The listing builds one solid part. Answer for the finished solid, in the listing's coordinates (mm). Round coordinates to 2 decimals unless told otherwise and drop trailing zeros. Loops run counter-clockwise (first coordinate to the right, second up) from the corner with the lowest first, then second, coordinate; pieces in that order, holes last. Notation, with made-up numbers: M 27.25,22 L 40.25,22 A13 ccw 40.25,47 Z; hole C 34,35 d7. An arc over 180 degrees is marked long. Put each result on its own line as item: value. Start each with the question number.
(1) Section A-A, the plane z = 2.45 is taken. Determine the outline of the cut face in (x, y), then the cut area to 3 significant figures.
(2) Section B-B, the plane y = 83 is taken. Determine the outline of the cut face in (x, z), then the cut area to 3 significant figures.
(3) Straight lines are drawn through the part: line 1 (Y direction, x = 0, z = 1); line 2 (X direction, y = -92, z = 0.85); line 3 (X direction, y = 65.5, z = 2.15). For each, find the intervals that lie inside material, in ascending order.
```python
from build123d import *

# Parameters (mm, degrees)
SKETCH1_W           = 439
SKETCH1_H           = 207
BOSS_EXTRUDE1_DEPTH = 3
FILLET1_R           = 40
CUT_EXTRUDE1_DEPTH  = 243.696312292
SKETCH3_R           = 1.6
CUT_EXTRUDE2_DEPTH  = 243.696312292
SKETCH4_R           = 1.6
CUT_EXTRUDE3_DEPTH  = 243.696312292


with BuildPart() as part:
    # Sketch1 → Boss-Extrude1 (new body)
    with BuildSketch(Plane.XY):
        Rectangle(SKETCH1_W, SKETCH1_H)
    extrude(amount=BOSS_EXTRUDE1_DEPTH)

    # Fillet1
    fillet1_edges = [part.edges().sort_by_distance(p)[0] for p in [
        (-219.5, 103.5, 1.5),
        (219.5, 103.5, 1.5),
    ]]
    fillet(fillet1_edges, radius=FILLET1_R)

    # Sketch2 → Cut-Extrude1 (cut, through all)
    with BuildSketch(Plane(origin=(0, 0, 0), x_dir=(-1, 0, 0), z_dir=(0, 0, -1))):
        with BuildLine():
            Line((-21, -83.5), (21, -83.5))
            ThreePointArc((21, -83.5), (24.535533906, -84.964466094), (26, -88.5))
            Line((26, -88.5), (26, -103.5))
            Line((26, -103.5), (-26, -103.5))
            Line((-26, -103.5), (-26, -88.5))
            ThreePointArc((-26, -88.5), (-24.535533906, -84.964466094), (-21, -83.5))
        make_face()
    extrude(amount=-CUT_EXTRUDE1_DEPTH, mode=Mode.SUBTRACT)

    # Sketch3 → Cut-Extrude2 (cut, through all)
    with BuildSketch(Plane.XY.offset(3)):
        with Locations((-207.5, 8.5)):
            Circle(SKETCH3_R)
        with Locations((207.5, 8.5)):
            Circle(SKETCH3_R)
    extrude(amount=-CUT_EXTRUDE2_DEPTH, mode=Mode.SUBTRACT)

    # Sketch4 → Cut-Extrude3 (cut, through all)
    with BuildSketch(Plane.XY.offset(3)):
        with Locations((0, 91.5)):
            Circle(SKETCH4_R)
    extrude(amount=-CUT_EXTRUDE3_DEPTH, mode=Mode.SUBTRACT)


solid = part.part
```
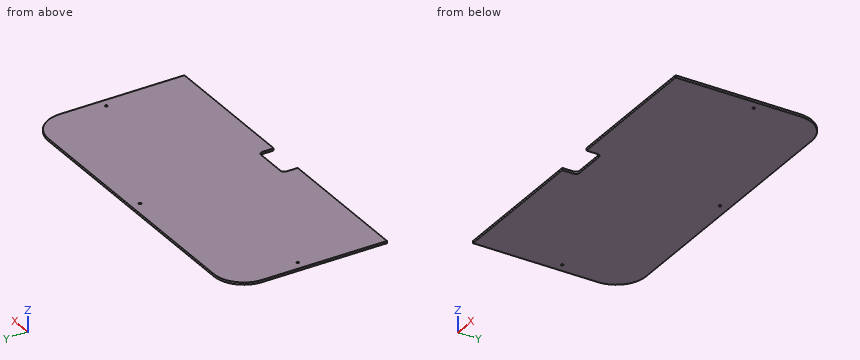
Recorded:
1. outline: M -219.5,-103.5 L -26,-103.5 L -26,-88.5 A5 cw -21,-83.5 L 21,-83.5 A5 cw 26,-88.5 L 26,-103.5 L 219.5,-103.5 L 219.5,63.5 A40 ccw 179.5,103.5 L -179.5,103.5 A40 ccw -219.5,63.5 Z; hole C -207.5,8.5 d3.2; hole C 0,91.5 d3.2; hole C 207.5,8.5 d3.2
1. area: 89,100 mm²
2. outline: M -214.42,0 L 214.42,0 L 214.42,3 L -214.42,3 Z
2. area: 1,290 mm²
3. line 1: y = -83.5 to 89.9, 93.1 to 103.5
3. line 2: x = -219.5 to -26, 26 to 219.5
3. line 3: x = -219.45 to 219.45
